```python
from build123d import *

# Parameters (mm, degrees)
SKETCH1_R           = 20
SKETCH1_R_2         = 2.55
BOSS_EXTRUDE1_DEPTH = 34
FILLET1_R           = 3


with BuildPart() as part:
    # Sketch1 → Boss-Extrude1 (new body)
    # profile 1 of 11: a face of its own
    with BuildSketch(Plane(origin=(0, 0, 0), x_dir=(0, 0, -1), z_dir=(1, 0, 0))):
        Circle(SKETCH1_R)
        with BuildLine():
            ThreePointArc((-15.415009376, -7.167809005), (-14.722431864, 8.5), (-1.5, 16.933694222))
            Line((-1.5, 16.933694222), (-1.5, 17))
            ThreePointArc((-1.5, 17), (0, 18.5), (1.5, 17))
            Line((1.5, 17), (1.5, 16.933694222))
            ThreePointArc((1.5, 16.933694222), (12.539936204, 11.478240283), (17, 0))
            ThreePointArc((17, 0), (16.599023456, -3.670479574), (15.415009376, -7.167809005))
            Line((15.415009376, -7.167809005), (15.472431864, -7.200961894))
            ThreePointArc((15.472431864, -7.200961894), (16.02146997, -9.25), (13.972431864, -9.799038106))
            Line((13.972431864, -9.799038106), (13.915009376, -9.765885217))
            ThreePointArc((13.915009376, -9.765885217), (0, -17), (-13.915009376, -9.765885217))
            Line((-13.915009376, -9.765885217), (-13.972431864, -9.799038106))
            ThreePointArc((-13.972431864, -9.799038106), (-16.02146997, -9.25), (-15.472431864, -7.200961894))
            Line((-15.472431864, -7.200961894), (-15.415009376, -7.167809005))
        make_face(mode=Mode.SUBTRACT)
    # profile 2 of 11: a face of its own
    with BuildSketch(Plane(origin=(0, 0, 0), x_dir=(0, 0, -1), z_dir=(1, 0, 0))):
        with BuildLine():
            ThreePointArc((1.486240766, 5.347297297), (0, 4.05), (-1.486240766, 5.347297297))
            ThreePointArc((-1.486240766, 5.347297297), (-4.806440991, 2.775), (-5.374015684, -1.386526389))
            ThreePointArc((-5.374015684, -1.386526389), (-3.507402885, -2.025), (-3.887774918, -3.960770908))
            ThreePointArc((-3.887774918, -3.960770908), (0, -5.55), (3.887774918, -3.960770908))
            ThreePointArc((3.887774918, -3.960770908), (3.507402885, -2.025), (5.374015684, -1.386526389))
            ThreePointArc((5.374015684, -1.386526389), (5.505828141, -0.698825069), (5.55, 0))
            ThreePointArc((5.55, 0), (4.418774505, 3.358114333), (1.486240766, 5.347297297))
        make_face()
        Circle(SKETCH1_R_2, mode=Mode.SUBTRACT)
    # profile 3 of 11: a face of its own
    with BuildSketch(Plane(origin=(0, 0, 0), x_dir=(0, 0, -1), z_dir=(1, 0, 0))):
        with BuildLine():
            ThreePointArc((-3.887774918, -3.960770908), (-3.507402885, -2.025), (-5.374015684, -1.386526389))
            ThreePointArc((-5.374015684, -1.386526389), (-4.806440991, -2.775), (-3.887774918, -3.960770908))
        make_face()
    # profile 4 of 11: a face of its own
    with BuildSketch(Plane(origin=(0, 0, 0), x_dir=(0, 0, -1), z_dir=(1, 0, 0))):
        with BuildLine():
            ThreePointArc((-13.915009376, -9.765885217), (-14.722431864, -8.5), (-15.415009376, -7.167809005))
            Line((-15.415009376, -7.167809005), (-15.472431864, -7.200961894))
            ThreePointArc((-15.472431864, -7.200961894), (-16.02146997, -9.25), (-13.972431864, -9.799038106))
            Line((-13.972431864, -9.799038106), (-13.915009376, -9.765885217))
        make_face()
    # profile 5 of 11: a face of its own
    with BuildSketch(Plane(origin=(0, 0, 0), x_dir=(0, 0, -1), z_dir=(1, 0, 0))):
        with BuildLine():
            ThreePointArc((3.887774918, -3.960770908), (4.806440991, -2.775), (5.374015684, -1.386526389))
            ThreePointArc((5.374015684, -1.386526389), (3.507402885, -2.025), (3.887774918, -3.960770908))
        make_face()
    # profile 6 of 11: a face of its own
    with BuildSketch(Plane(origin=(0, 0, 0), x_dir=(0, 0, -1), z_dir=(1, 0, 0))):
        with BuildLine():
            ThreePointArc((1.486240766, 5.347297297), (0, 5.55), (-1.486240766, 5.347297297))
            ThreePointArc((-1.486240766, 5.347297297), (0, 4.05), (1.486240766, 5.347297297))
        make_face()
    # profile 7 of 11: a face of its own
    with BuildSketch(Plane(origin=(0, 0, 0), x_dir=(0, 0, -1), z_dir=(1, 0, 0))):
        with BuildLine():
            Line((15.472431864, -7.200961894), (15.415009376, -7.167809005))
            ThreePointArc((15.415009376, -7.167809005), (14.722431864, -8.5), (13.915009376, -9.765885217))
            Line((13.915009376, -9.765885217), (13.972431864, -9.799038106))
            ThreePointArc((13.972431864, -9.799038106), (16.02146997, -9.25), (15.472431864, -7.200961894))
        make_face()
    # profile 8 of 11: a face of its own
    with BuildSketch(Plane(origin=(0, 0, 0), x_dir=(0, 0, -1), z_dir=(1, 0, 0))):
        with BuildLine():
            ThreePointArc((13.915009376, -9.765885217), (14.722431864, -8.5), (15.415009376, -7.167809005))
            Line((15.415009376, -7.167809005), (5.556440991, -1.475961894))
            ThreePointArc((5.556440991, -1.475961894), (5.466744289, -1.428151993), (5.374015684, -1.386526389))
            ThreePointArc((5.374015684, -1.386526389), (4.806440991, -2.775), (3.887774918, -3.960770908))
            ThreePointArc((3.887774918, -3.960770908), (3.970188051, -4.020263434), (4.056440991, -4.074038106))
            Line((4.056440991, -4.074038106), (13.915009376, -9.765885217))
        make_face()
    # profile 9 of 11: a face of its own
    with BuildSketch(Plane(origin=(0, 0, 0), x_dir=(0, 0, -1), z_dir=(1, 0, 0))):
        with BuildLine():
            Line((-5.556440991, -1.475961894), (-15.415009376, -7.167809005))
            ThreePointArc((-15.415009376, -7.167809005), (-14.722431864, -8.5), (-13.915009376, -9.765885217))
            Line((-13.915009376, -9.765885217), (-4.056440991, -4.074038106))
            ThreePointArc((-4.056440991, -4.074038106), (-3.970188051, -4.020263434), (-3.887774918, -3.960770908))
            ThreePointArc((-3.887774918, -3.960770908), (-4.806440991, -2.775), (-5.374015684, -1.386526389))
            ThreePointArc((-5.374015684, -1.386526389), (-5.466744289, -1.428151993), (-5.556440991, -1.475961894))
        make_face()
    # profile 10 of 11: a face of its own
    with BuildSketch(Plane(origin=(0, 0, 0), x_dir=(0, 0, -1), z_dir=(1, 0, 0))):
        with BuildLine():
            Line((-1.5, 16.933694222), (-1.5, 5.55))
            ThreePointArc((-1.5, 5.55), (-1.496556238, 5.448415427), (-1.486240766, 5.347297297))
            ThreePointArc((-1.486240766, 5.347297297), (0, 5.55), (1.486240766, 5.347297297))
            ThreePointArc((1.486240766, 5.347297297), (1.496556238, 5.448415427), (1.5, 5.55))
            Line((1.5, 5.55), (1.5, 16.933694222))
            ThreePointArc((1.5, 16.933694222), (0, 17), (-1.5, 16.933694222))
        make_face()
    # profile 11 of 11: a face of its own
    with BuildSketch(Plane(origin=(0, 0, 0), x_dir=(0, 0, -1), z_dir=(1, 0, 0))):
        with BuildLine():
            Line((-1.5, 17), (-1.5, 16.933694222))
            ThreePointArc((-1.5, 16.933694222), (0, 17), (1.5, 16.933694222))
            Line((1.5, 16.933694222), (1.5, 17))
            ThreePointArc((1.5, 17), (0, 18.5), (-1.5, 17))
        make_face()
    extrude(amount=BOSS_EXTRUDE1_DEPTH)

    # Fillet1
    fillet1_edges = [part.edges().sort_by_distance(p)[0] for p in [
        (17, 16.933694222, -1.5),
        (17, 5.347297297, -1.486240766),
        (17, 5.347297297, 1.486240766),
        (17, -1.386526389, -5.374015684),
        (17, -3.960770908, -3.887774918),
        (17, -7.167809005, -15.415009376),
        (17, -3.960770908, 3.887774918),
        (17, -1.386526389, 5.374015684),
        (17, -9.765885217, 13.915009376),
        (17, -9.765885217, -13.915009376),
        (17, 16.933694222, 1.5),
        (17, -7.167809005, 15.415009376),
    ]]
    fillet(fillet1_edges, radius=FILLET1_R)


solid = part.part
```
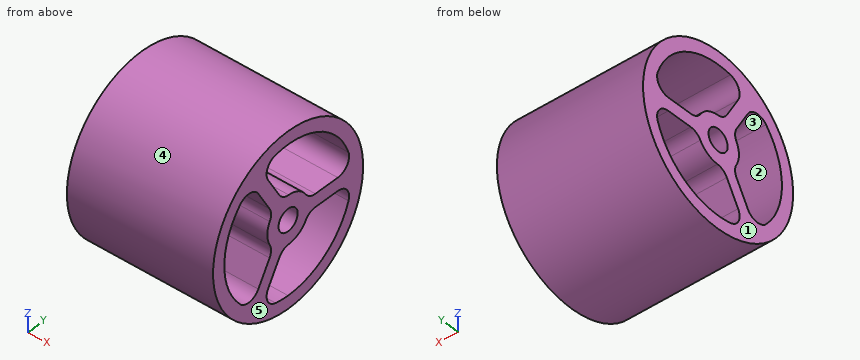
Can you work these out from the model? Positions are in its coordinate system, mm. Face numbers are marked on the shaded views. A direction names the side the tool comes from. Round coordinates to 2 decimals unless told otherwise and drop trailing zeros. Loops run counter-clockwise (first coordinate to the right, second up) from the corner with the lowest first, then second, coordinate; pieces in that order, holes last. Notation, with made-up numbers: (-4.75, -27.5) -> (41.25, -27.5) arc R21 ccw to (41.25, 9.5) -> close; hole circle Ø3 at (85, 82). An arc over 180 degrees is marked (long way). Answer in a Markdown table with one row per item.
Item 1: If I drill on probe 1 along Y at (x, z) = (10, 0); probe 2 along Z at (x, y) = (18.5, 13); probe 3 along Y at (x, z) = (2, 3), over which ranges is the centre line in solid material (lowest first)?
Answer block:
| item | result |
|---|---|
| probe 1 | -20 to -17, -5.55 to -2.55, 2.55 to 20 |
| probe 2 | -15.2 to -10.95, -1.5 to 1.5, 10.95 to 15.2 |
| probe 3 | -19.77 to -16.73, -4.72 to 4.67, 15.86 to 19.77 |
Item 2: Will these pins go through, and if not, where does the flat tip stop? P1, Ø1.5, axis at x = 17, z = -1, coming from the +Y side; P2, Ø6.5, axis at x = 21.5, y = 11, coming from the -Z side; P3, Ø5, axis at x = 25.5, y = -13, coming from the +Z side; P4, Ø4, axis at y = 0, z = 0, coming from the -X side.
Answer block:
| item | result |
|---|---|
| P1 | y = 20 |
| P2 | z = -18.44 |
| P3 | z = 17.02 |
| P4 | through |
Item 3: We'd pull the mould along Z, two halves only. Please class the marked faces 3, 4 and 5: released by +Z, released by -Z, zero draft, split by the parting line, or undercut.
Answer block:
| item | result |
|---|---|
| face 3 | undercut |
| face 4 | split by the parting line |
| face 5 | zero draft |
Item 4: Suppose I cut it at D-D, the plane x = 14. Give the number of separate pieces and of enclosed holes in the cut face, plus the area to 3 significant figures.
Answer block:
| item | result |
|---|---|
| separate pieces | 1 |
| enclosed holes | 4 |
| area | 552 mm² |
Item 5: Suppose I cut it at A-A, the plane z = 0. List the corners of the cut face in (x, y) for me, plus the area to 3 significant figures.
Answer block:
| item | result |
|---|---|
| outline | (0, -20) -> (34, -20) -> (34, -17) -> (0, -17) -> close; (0, -5.55) -> (34, -5.55) -> (34, -2.55) -> (0, -2.55) -> close; (0, 2.55) -> (34, 2.55) -> (34, 20) -> (0, 20) -> close |
| area | 797 mm² |
Item 6: Suppose I cut it at C-C, the plane y = -8.5. List the corners of the cut face in (x, z) for me.
Answer block:
| item | result |
|---|---|
| outline | (0, -18.1) -> (34, -18.1) -> (34, -11.44) -> (0, -11.44) -> close; (0, 11.44) -> (34, 11.44) -> (34, 18.1) -> (0, 18.1) -> close |
Item 7: Suppose I cut it at B-B, the plane y = 12.5. List the corners of the cut face in (x, z) for me.
Answer block:
| item | result |
|---|---|
| outline | (0, -15.61) -> (34, -15.61) -> (34, -11.52) -> (0, -11.52) -> close; (0, -1.5) -> (34, -1.5) -> (34, 1.5) -> (0, 1.5) -> close; (0, 11.52) -> (34, 11.52) -> (34, 15.61) -> (0, 15.61) -> close |
Item 8: On a 3-axis mill with a long thin cutter (end or side, diameter ignored), from which of +Z, -Z, +X, -X, +Y, -Y can I reach the whole of each face in a straight line? I mean the marked faces 1 and 2. Say none if no direction works.
Answer block:
| item | result |
|---|---|
| face 1 | +Z, -Z, -X, +Y, -Y |
| face 2 | +X, -X |
